from build123d import *

# Parameters (mm, degrees)
AXIAL_HOLES_DEPTH      = 193.994533601
AXIAL_HOLES_DEPTH_BACK = 193.994533601
SKETCH2_R              = 1.65
CUT_EXTRUDE2_START     = 135.7
SKETCH3_R              = 2.85
CUT_EXTRUDE2_DEPTH     = 4


with BuildPart() as part:
    # Axial profile (mm) → Full revolution (revolve)
    with BuildSketch(Plane.XY, mode=Mode.PRIVATE) as full_revolution_sk:
        Polygon((135.7, 36.4), (179.7, 36.4), (179.7, 23.4), (181.7, 23.4), (181.7, 39), (139.7, 39), (139.7, 46), (135.7, 46), align=None)
    revolve(full_revolution_sk.sketch.rotate(Axis((-110, 0, 0), (1, 0, 0)), 90), axis=Axis((-110, 0, 0), (1, 0, 0)))

    # Sketch2 → Axial holes (cut, two sides: drawn at the far end of the back side and taken through both)
    with BuildSketch(Plane(origin=(0, 0, 0), x_dir=(0, 0, -1), z_dir=(1, 0, 0)).offset(-AXIAL_HOLES_DEPTH_BACK)):
        with Locations(Location((0, 42.2, 0), (0, 0, 180))):
            Circle(SKETCH2_R)
        with Locations(Location((-36.54627204, -21.1, 0), (0, 0, 180))):
            Circle(SKETCH2_R)
        with Locations(Location((36.54627204, -21.1, 0), (0, 0, 180))):
            Circle(SKETCH2_R)
    extrude(amount=AXIAL_HOLES_DEPTH + AXIAL_HOLES_DEPTH_BACK, mode=Mode.SUBTRACT)

    # Sketch3 → Cut-Extrude2 (cut)
    with BuildSketch(Plane(origin=(0, 0, 0), x_dir=(0, 0, -1), z_dir=(1, 0, 0)).offset(CUT_EXTRUDE2_START)):
        with Locations((0, 42.2)):
            Circle(SKETCH3_R)
        with Locations((-36.54627204, -21.1)):
            Circle(SKETCH3_R)
        with Locations((36.54627204, -21.1)):
            Circle(SKETCH3_R)
    extrude(amount=CUT_EXTRUDE2_DEPTH, mode=Mode.SUBTRACT)


solid = part.part
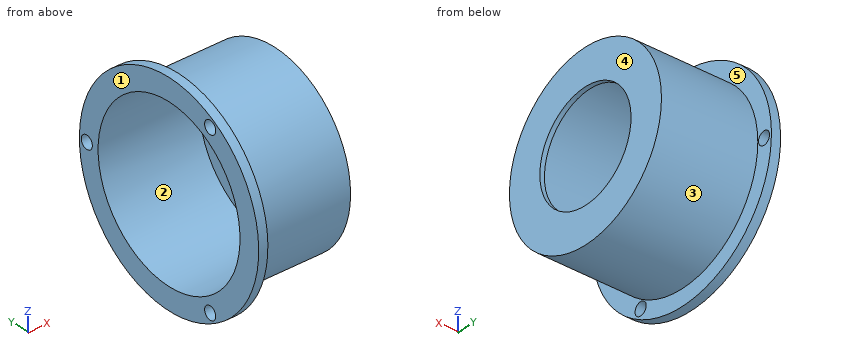
Work out the finished part from the listing and answer in its coordinate system (mm). Face numbers are marked on the shaded views. A direction names the side the tool comes from. Give positions to 0.01 mm unless a question says otherwise; leave off trailing zeros. Order: outer loops, then holes, each group sorted by start corner. A loop starts at its lowest first (then second) coordinate and runs counter-clockwise, first axis right, second up. Notation, with made-up numbers: (19, 81) -> (52, 81) arc R18 ccw to (52, 105) -> close; hole circle Ø7 at (-36.5, 57). An arc over 180 degrees is marked (long way). Answer as a JSON object with one key per item and string values. Group by question number.
1. Section B-B on z = 11 is taken. Determine the outline of the cut face in (x, y), plus the area to 3 significant figures.
2. Flat-ended cylindrical pins translate along their axes: pin 1 Ø6.5 at (y, z) = (-21.1, 36.55) entering from +X; pin 2 Ø4 at (x, y) = (153, -29) entering from +Z; pin 3 Ø12 at (y, z) = (-16, -23) entering from -X; pin 4 Ø1 at (x, z) = (143.5, 23.5) entering from +Y. Find the tip coordinate at first contact, or state that the pin passes through.
3. Consider line 1 along Y through (x, z) = (138.2, 0); line 2 along Y through (x, z) = (180, 0); line 3 along X through (y, z) = (-19, -41). Determine where each line is inside the solid, lowest interval first. Write a range as [from, to].
4. Section A-A on y = 0 is taken. Determine the outline of the cut face in (x, z), plus the area to 3 significant figures.
5. Section C-C on y = -21.1 is taken. Determine the outline of the cut face in (x, z), plus the area to 3 significant figures.
6. Section D-D on x = 142.5 is taken. Determine the outline of the cut face in (y, z), plus the area to 3 significant figures.
7. A tool of negligible diameter and unlimited length cuts with its end or side. For the marked faces 4 and 5, from which of +Z, -Z, +X, -X, +Y, -Y can it reach the whole face along a straight path? Write none if from no direction.
8. The mould has two halves that part along Z. Classify the marked faces 1, 2 and 3: released by +Z, released by -Z, zero draft, split by the parting line, or undercut.
Result sheet:
{
 "1": {"outline": "(135.7, -44.67) -> (139.7, -44.67) -> (139.7, -37.42) -> (181.7, -37.42) -> (181.7, -20.65) -> (179.7, -20.65) -> (179.7, -34.7) -> (135.7, -34.7) -> close; (135.7, 34.7) -> (179.7, 34.7) -> (179.7, 20.65) -> (181.7, 20.65) -> (181.7, 37.42) -> (139.7, 37.42) -> (139.7, 44.67) -> (135.7, 44.67) -> close", "area": "364 mm^2"},
 "2": {"pin 1": "stops at x = 181.7", "pin 2": "stops at z = 28.14", "pin 3": "stops at x = 179.7", "pin 4": "stops at y = 31.5"},
 "3": {"line 1": "y = [-46, -36.4], [36.4, 39.35], [45.05, 46]", "line 2": "y = [-39, -23.4], [23.4, 39]", "line 3": "x = [135.7, 139.7]"},
 "4": {"outline": "(135.7, -46) -> (139.7, -46) -> (139.7, -39) -> (181.7, -39) -> (181.7, -23.4) -> (179.7, -23.4) -> (179.7, -36.4) -> (135.7, -36.4) -> close; (135.7, 36.4) -> (179.7, 36.4) -> (179.7, 23.4) -> (181.7, 23.4) -> (181.7, 39) -> (139.7, 39) -> (139.7, 46) -> (135.7, 46) -> close", "area": "347 mm^2"},
 "5": {"outline": "(135.7, -40.88) -> (139.7, -40.88) -> (139.7, -39.4) -> (135.7, -39.4) -> close; (135.7, -33.7) -> (139.7, -33.7) -> (139.7, -32.8) -> (181.7, -32.8) -> (181.7, -10.12) -> (179.7, -10.12) -> (179.7, -29.66) -> (135.7, -29.66) -> close; (135.7, 29.66) -> (179.7, 29.66) -> (179.7, 10.12) -> (181.7, 10.12) -> (181.7, 32.8) -> (139.7, 32.8) -> (139.7, 33.7) -> (135.7, 33.7) -> close; (135.7, 39.4) -> (139.7, 39.4) -> (139.7, 40.88) -> (135.7, 40.88) -> close", "area": "386 mm^2"},
 "6": {"outline": "circle Ø78 at (0, 0); hole circle Ø72.8 at (0, 0)", "area": "616 mm^2"},
 "7": {"face 4": "+Z, -Z, +X, +Y, -Y", "face 5": "+X"},
 "8": {"face 1": "zero draft", "face 2": "undercut", "face 3": "split by the parting line"}
}
